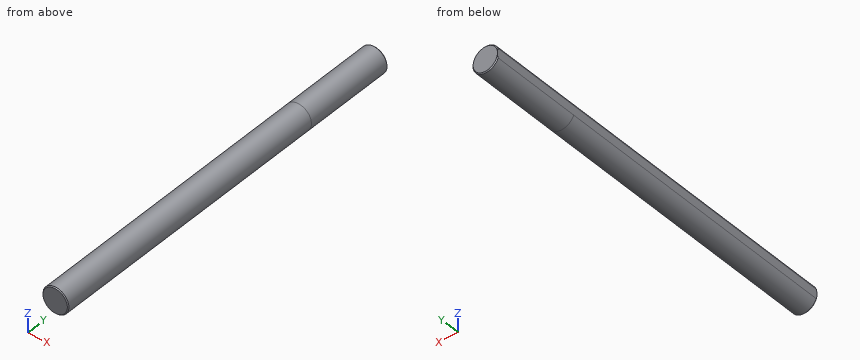
Autodesk Inventor part; units mm, degrees
ref_plane "Work Plane1" through (0, 72.5, 0) normal (0, 1, 0) x (1, 0, 0)
ref_plane "Work Plane2" through (-7.5, 0, 0) normal (1, 0, 0) x (0, 1, 0)
ref_plane "Work Plane3" through (0, 27.5, 0) normal (0, -1, 0) x (1, 0, 0)
sketch "Sketch1" plane through (0, 0, 0) normal (0, 1, 0) x (-1, 0, 0)
  circle A0 centre (0, 0) radius 7.5
  dimension "d0" = 15
extrude "Extrusion1" add sketch "Sketch1" along normal blind 100
ref_plane "Work Plane1" through (0, 72.5, 0) normal (0, 1, 0) x (1, 0, 0)
sketch "Sketch2" plane through (0, 72.5, 0) normal (0, 1, 0) x (1, 0, 0)
  circle A0 centre (0, 0) radius 7.5
ref_plane "Work Plane2" through (-7.5, 0, 0) normal (1, 0, 0) x (0, 1, 0)
ref_plane "Work Plane3" through (0, 27.5, 0) normal (0, -1, 0) x (1, 0, 0)
sketch "Sketch3" plane through (-7.5, 0, 0) normal (1, 0, 0) x (0, 1, 0)
  line L0 (27.5, -10.5) -> (27.5, 10.5)
  line L1 (72.5, 10.5) -> (72.5, -10.5)
  line L2 (0, -7.5) -> (0, 7.5)
  line L3 (27.5, -3) -> (0, -3)
  line L4 (0, -3) -> (0, 3)
  line L5 (0, 3) -> (27.5, 3)
  line L6 (27.5, 3) -> (27.5, -3)
  line L7 (100, -7.5) -> (100, 7.5)
  line L8 (72.5, -3) -> (100, -3)
  line L9 (100, -3) -> (100, 3)
  line L10 (100, 3) -> (72.5, 3)
  line L11 (72.5, 3) -> (72.5, -3)
  line L12 (27.5, -3) -> (72.5, -3)
  line L13 (72.5, -3) -> (72.5, 3)
  line L14 (72.5, 3) -> (27.5, 3)
  line L15 (27.5, 3) -> (27.5, -3)
  point P0 (0, 0)
extrude "Extrusion3" cut sketch "Sketch3" along normal blind 0.5 contours L0 L14 L1 L12 | L1 L10 L7 L8
extrude "Extrusion2" [suppressed]
chamfer "Chamfer1" [suppressed]
sketch "Sketch4" plane through (0, 0, 0) normal (0, -1, 0) x (1, 0, 0)
  circle A0 centre (0, 0) radius 7.5
  circle A1 centre (0, 0) radius 7.5
extrude "Extrusion4" add sketch "Sketch4" along normal blind 67.5
sketch "Sketch5" plane through (0, 100, 0) normal (0, 1, 0) x (1, 0, 0)
  arc A0 (-7, -2.6926) -> (-7, 2.6926) centre (0, 0) ccw
  line L0 (-7, 2.6926) -> (-7, -2.6926)
  arc A1 (-7, -2.6926) -> (-7, 2.6926) centre (0, 0) ccw
  point P0 (-7, 2.6926)
extrude "Extrusion5" add sketch "Sketch5" along normal blind 52.5
sketch "Sketch6" plane through (-7, 0, 0) normal (-1, 0, 0) x (0, 0, 1)
  line L0 (-2.6926, 27.5) -> (-2.6926, 152.5)
  line L1 (2.6926, 152.5) -> (2.6926, 27.5)
  line L2 (-2.6926, 152.5) -> (2.6926, 152.5)
  line L3 (-2.6926, 152.5) -> (2.6926, 152.5)
  line L4 (0, 152.5) -> (0, 72.5)
  line L5 (0, 152.5) -> (80, 152.5) construction
  circle A0 centre (0, 72.5) radius 1.25
  circle A1 centre (0, 72.5) radius 0.75
  circle A2 centre (0, 72.5) radius 0.75
  line L6 (-7.5, -67.5) -> (7.5, -67.5)
  line L7 (-2.6926, 26.1771) -> (2.6926, 26.1771)
  line L8 (2.6926, 26.1771) -> (2.6926, -67.5)
  line L9 (2.6926, -67.5) -> (-2.6926, -67.5)
  line L10 (-2.6926, -67.5) -> (-2.6926, 26.1771)
  line L11 (2.6926, 27.5) -> (-2.6926, 27.5)
  line L12 (2.6926, 26.1771) -> (2.6926, 27.5)
  line L13 (-2.6926, 27.5) -> (-2.6926, 152.5)
  line L14 (-2.6926, 26.1771) -> (-2.6926, 27.5)
  point P0 (0, 0)
  dimension "d23" = 80
  dimension "d24" = 90
  dimension "d25" = 2.5
  dimension "d26" = 1.5
extrude "Extrusion6" [suppressed]
chamfer "Chamfer3" [suppressed]
extrude "Extrusion7" cut sketch "Sketch6" along normal blind 0.5 contours L11 L12 L7 L14 | L7 L8 L6 L10
chamfer "Chamfer4" distance 0.5 angle 45 2 edges at (7.5, 152.5, 0) (7.5, -67.5, 0)
properties part number "wał_uzębienia" material "Stainless Steel"
Can you work these out from the model? Positions are in its coordinate system, mm. Round coordinates to 2 decimals unless told otherwise and drop trailing zeros. Loops run counter-clockwise (first coordinate to the right, second up) from the corner with the lowest first, then second, coordinate; pieces in that order, holes last. Notation, with made-up numbers: M -25.75,14.5 L 12.25,14.5 A19 ccw 12.25,36.5 Z; hole C -29.75,89 d1. An arc over 180 degrees is marked long. Write item = value, one per line. Start each with the question number.
(1) I need wall thicknesses on line 1 along Z through (x, y) = (0.5, 93.5); line 2 along X through (y, z) = (138, 0.5); line 3 along X through (y, z) = (113, 1.75). Which ranges of each line are inside material? Lowest first, please.
(2) I'm going to push flat-ended pins straight in: P1, Ø5, axis at x = -5, y = 51, coming from the -Z side; P2, Ø2, axis at x = -4.5, y = 103.5, coming from the +Z side; P3, Ø8, axis at y = 76.5, z = 5.5, coming from the +X side. Where does each tip first touch, or does it pass through?
(3) Suppose I cut it at A-A on y = 56. Write out the boundary of the cut face in (x, z), plus the area to 3 significant figures.
Answer block:
q1.line_1 = -7.48 to 7.48
q1.line_2 = -7 to 7.48
q1.line_3 = -7 to 7.29
q2.P1 = -7.07
q2.P2 = 6.63
q2.P3 = 7.35
q3.outline = M -7,-2.69 A7.5 ccw long -7,2.69 Z
q3.area = 175 mm²
